Part model, mm, in its own coordinate system. Face numbers are marked on the shaded views. A direction names the side the tool comes from. Round coordinates to 2 decimals unless told otherwise and drop trailing zeros. Write each loop counter-clockwise with the first axis right and the second up, starting at its lowest first coordinate (ties: lowest second). Pieces come first, ordered by that corner, then holes.
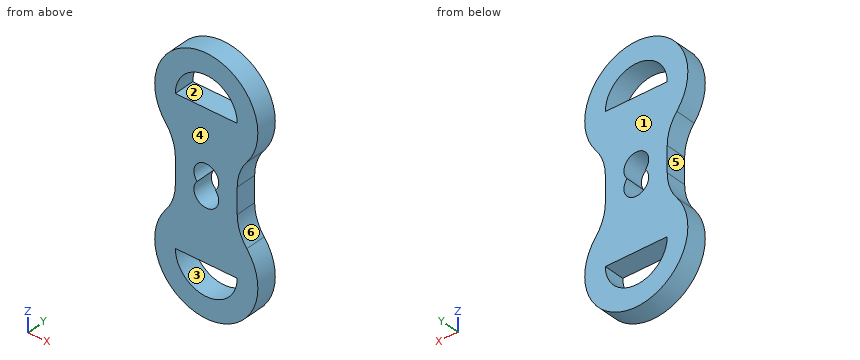
Autodesk Inventor part; units mm, degrees
ref_plane "YZ Plane" through (0, 0, 0) normal (1, 0, 0) x (0, 1, 0)
ref_plane "XZ Plane" through (0, 0, 0) normal (0, 1, 0) x (-1, 0, 0)
ref_plane "XY Plane" through (0, 0, 0) normal (0, 0, 1) x (1, 0, 0)
sketch "Boceto1" plane through (0, 0, 0) normal (0, 1, 0) x (-1, 0, 0)
  line L0 (0, 35) -> (0, -35) construction
  arc A0 (25, 35) -> (-25, 35) centre (0, 35) ccw
  arc A1 (-25, -35) -> (25, -35) centre (0, -35) ccw
  circle A2 centre (0, -35) radius 15
  circle A3 centre (0, 35) radius 15
  line L1 (0, -20) -> (0, -20)
  line L2 (15, -35) -> (-15, -35)
  line L3 (94.5074, 0) -> (-76.0102, 0) construction
  line L4 (15, 35) -> (-15, 35)
  line L5 (15, -35) -> (-15, -35)
  line L6 (15, -6.1794) -> (-15, -6.1794)
  line L7 (-15, -6.1794) -> (-15, 6.1794)
  line L8 (-15, 6.1794) -> (15, 6.1794)
  line L9 (15, 6.1794) -> (15, -6.1794)
  line L10 (15, -6.1794) -> (-15, 6.1794) construction
  line L11 (-15, -6.1794) -> (15, 6.1794) construction
  circle A4 centre (0, -35) radius 25
  arc A5 (15, -6.1794) -> (19.6273, -19.5155) centre (36.5312, -6.1794) ccw
  line L12 (0, -66.9543) -> (0, 90.1933) construction
  arc A6 (-19.6273, -19.5155) -> (-15, -6.1794) centre (-36.5312, -6.1794) ccw
  circle A7 centre (0, 35) radius 25
  arc A8 (19.6273, 19.5155) -> (15, 6.1794) centre (36.5312, 6.1794) ccw
  arc A9 (-15, 6.1794) -> (-19.6273, 19.5155) centre (-36.5312, 6.1794) ccw
  circle A10 centre (0, 4) radius 6
  circle A11 centre (0, -4) radius 6
  point P0 (0, 0)
  point P1 (0, 60)
  point P2 (0, -60)
  point P3 (0, -20)
  point P4 (15, 35)
  point P5 (0, 0)
  point P6 (15, 6.1794)
  point P7 (25, 35)
  point P8 (-25, 35)
  point P9 (-19.6273, 19.5155)
  point P10 (-15, 6.1794)
  point P11 (-12.5, -0.1825)
  point P12 (-19.6273, -19.5155)
  point P13 (25, -35)
  point P14 (-15, 6.1794)
  point P15 (4.4721, 0)
  point P16 (-4.4721, 0)
  dimension "largo" = 120
  dimension "espesor_junta" = 10
  dimension "d3" = 10
  dimension "d6" = 0
  dimension "d29" = 30
  dimension "d35" = 12
  dimension "d36" = 12
  dimension "d37" = 8
  dimension "d38" = 4
extrude "Extrusión8" add sketch "Boceto1" along normal blind 10 contours A7 A0 | A8 L8 A10 A7 | A7 A10 L8 A9 | L9 L6 A11 A10 L8 | L8 A10 A11 L6 L7 | A5 A4 A11 L6 | L6 A11 A4 A6 | A4 A1 | L2 A2 | A3 L4 picked at (1.773, -30.3249) picked at (0.6027, 30.0365)
equation "\"d3\" = espesor_junta"
properties part number "mod5" material "Aluminio 6061"
Q1. Mould opens along Z. For the marked faces 1 and 2 say: +Z half, -Z half, draft (parallel to the pull), parting line (faces both ways), or undercut.
Values follow:
face 1: draft
face 2: undercut
Q2. Cut at D-D on y = 6.75. Write the cut outline in (x, z).
Values follow:
outline: (-19.63, -19.52) arc R25 ccw (long way) to (19.63, -19.52) arc R21.53 cw to (15, -6.18) - (15, 6.18) arc R21.53 cw to (19.63, 19.52) arc R25 ccw (long way) to (-19.63, 19.52) arc R21.53 cw to (-15, 6.18) - (-15, -6.18) arc R21.53 cw to start; hole (-15, -35) arc R15 ccw to (15, -35) - close; hole (-15, 35) - (15, 35) arc R15 ccw to start; hole (-4.47, 0) arc R6 ccw (long way) to (4.47, 0) arc R6 ccw (long way) to start
Q3. Wall check: L1, parallel to Z at x = 0, y = 3.75; L2, parallel to Z at x = 11.5, y = 5; L3, parallel to Z at x = -7, y = 4.5. Give the ranges that are in metal, low to high.
Values follow:
L1: z = -60 to -50, -35 to -10, 10 to 35, 50 to 60
L2: z = -57.2 to -44.63, -35 to 35, 44.63 to 57.2
L3: z = -59 to -48.27, -35 to 35, 48.27 to 59
Q4. Cut at A-A on x = 0. Write the cut outline in (y, z), plus the area to 3 significant figures.
Values follow:
outline: (0, -60) - (10, -60) - (10, -50) - (0, -50) - close; (0, -35) - (10, -35) - (10, -10) - (0, -10) - close; (0, 10) - (10, 10) - (10, 35) - (0, 35) - close; (0, 50) - (10, 50) - (10, 60) - (0, 60) - close
area: 700 mm2
Q5. Which spindle directions (+Z, -Z, +X, -X, +Y, -Y) get a long thin tool onto all of the face, cutting with end or side? Do the marked faces 3, 4, 5 and 6. Say none if no direction does.
Values follow:
face 3: +Y, -Y
face 4: +Z, -Z, +X, -X, -Y
face 5: -X, +Y, -Y
face 6: +X, +Y, -Y
Q6. Drop flat-ended pins along their axis: pin 1 (2 mm diameter, centred on x = 12, y = 3.5, fed in from -Z); pin 2 (6 mm diameter, centred on y = 6, z = -28, fed in from +X); pin 3 (3 mm diameter, centred on y = 4, z = 2.5, fed in from -X). Give the stop position or say it passes through.
Values follow:
pin 1: stops at z = -57.45
pin 2: stops at x = 24.68
pin 3: stops at x = -15
Q7. Cut at B-B on z = 4. Write the cut outline in (x, y).
Values follow:
outline: (-15, 0) - (-6, 0) - (-6, 10) - (-15, 10) - close; (6, 0) - (15, 0) - (15, 10) - (6, 10) - close
Q8. Cut at C-C on x = -7.5. Write the cut outline in (y, z).
Values follow:
outline: (0, -58.85) - (10, -58.85) - (10, -47.99) - (0, -47.99) - close; (0, -35) - (10, -35) - (10, 35) - (0, 35) - close; (0, 47.99) - (10, 47.99) - (10, 58.85) - (0, 58.85) - close
